```python
from build123d import *

# Parameters (mm, degrees)
F0_W     = 400
F0_H     = 26
F1_DEPTH = 38
F2_T     = -1.5
F3_W     = 38
F3_H     = 1.5
F4_DEPTH = 12
F5_W     = 38
F5_H     = 1.5
F6_DEPTH = 12
F7_R     = 2.5
F8_DEPTH = 1.5
F9_R     = 3


with BuildPart() as f1:
    # F0 (on Front) → F1 (new body)
    with BuildSketch(Plane.XZ):
        with Locations((200, 13)):
            Rectangle(F0_W, F0_H)
    extrude(amount=-F1_DEPTH)

    # F2
    f2_openings = [f1.faces().sort_by_distance(p)[0] for p in [
        (200, 19, 26),
        (200, 38, 13),
    ]]
    offset(amount=F2_T, openings=f2_openings)

    # F3 (on face) → F4 (join)
    with BuildSketch(Plane.YZ.offset(400)):
        with Locations((19, 25.25)):
            Rectangle(F3_W, F3_H)
    extrude(amount=F4_DEPTH)

    # F5 (on face) → F6 (join)
    with BuildSketch(Plane(origin=(0, 0, 0), x_dir=(0, -1, 0), z_dir=(-1, 0, 0))):
        with Locations((-19, 25.25)):
            Rectangle(F5_W, F5_H)
    extrude(amount=F6_DEPTH)

    # F7 (on face) → F8 (cut, through all)
    with BuildSketch(Plane.XY.offset(26)):
        with Locations((405.75, 7.5)):
            Circle(F7_R)
        with Locations((-5.75, 7.5)):
            Circle(F7_R)
    extrude(amount=-F8_DEPTH, mode=Mode.SUBTRACT)

    # F9
    f9_edges = [f1.edges().sort_by_distance(p)[0] for p in [
        (-12, 0, 25.25),
        (-12, 38, 25.25),
        (412, 0, 25.25),
        (412, 38, 25.25),
    ]]
    fillet(f9_edges, radius=F9_R)


solid = f1.part
```
Geometry: final body of the model. Coordinates: model frame, mm. A direction names the side the tool comes from. Give positions to 0.01 mm unless a question says otherwise; leave off trailing zeros. Write each loop counter-clockwise with the first axis right and the second up, starting at its lowest first coordinate (ties: lowest second). Pieces come first, ordered by that corner, then holes.
1. Draft query along X for faces 4 (the flat face through (1.5, 19, 14)), 5 (the flat face through (203, 0, 13)), 6 (the flat face through (197, 1.5, 14)), 7 (the flat face through (400, 19, 12)). Return one class per face: released by +X, released by -X, zero draft, split by the parting line, or undercut.
2. Section query A-A, the plane y = 20. Return loops of the section in (x, z), then the cut area to 4 significant figures.
3. Pin query (flat end, axial travel): P1, Ø3, axis at x = 263.5, z = 11, coming from the -Y side; P2, Ø3, axis at y = 9.5, z = 4, coming from the -X side; P3, Ø5, axis at x = 311, z = 15.5, coming from the +Y side; P4, Ø6, axis at x = 407.5, y = 22.5, coming from the -Z side. Return the tip coordinate at first contact, or that it passes through.
4. Reachability of faces 1 (the flat face through (197, 19, 1.5)), 2 (the flat face through (406, 19, 24.5)), 3 (the flat face through (0, 19, 12)) from +Z, -Z, +X, -X, +Y, -Y: full face, straight path, thin tool, end or side. Return the list, or none.
5. Section query B-B, the plane x = 216. Return loops of the section in (y, z).
6. Section query C-C, the plane z = 12.75. Return loops of the section in (x, y).
7. Line query: probe 1 along X at (y, z) = (14.5, 6.25); probe 2 along Y at (x, z) = (405.75, 25.55); probe 3 along Z at (x, y) = (85.5, 19). Output: solid intervals per line, ascending.
Computed:
1. face 4: undercut
1. face 5: zero draft
1. face 6: undercut
1. face 7: released by +X
2. outline: (-12, 24.5) - (0, 24.5) - (0, 0) - (400, 0) - (400, 24.5) - (412, 24.5) - (412, 26) - (398.5, 26) - (398.5, 1.5) - (1.5, 1.5) - (1.5, 26) - (-12, 26) - close
2. area: 709.5 mm2
3. P1: stops at y = 0
3. P2: stops at x = 0
3. P3: stops at y = 1.5
3. P4: stops at z = 24.5
4. face 1: +Z, +Y
4. face 2: -Z, +X, +Y, -Y
4. face 3: -Z, -X, +Y, -Y
5. outline: (0, 0) - (38, 0) - (38, 1.5) - (1.5, 1.5) - (1.5, 26) - (0, 26) - close
6. outline: (0, 0) - (400, 0) - (400, 38) - (398.5, 38) - (398.5, 1.5) - (1.5, 1.5) - (1.5, 38) - (0, 38) - close
7. probe 1: x = 0 to 1.5, 398.5 to 400
7. probe 2: y = 0 to 5, 10 to 38
7. probe 3: z = 0 to 1.5
